from build123d import *

# Parameters (mm, degrees)
F0_R     = 2.3495
F0_R_2   = 9.525
F0_R_3   = 12.7
F0_R_4   = 2.0955
F0_R_5   = 10.9855
F1_DEPTH = 5
F2_R     = 19.05
F3_DEPTH = 5.08


with BuildPart() as f1:
    # F0 (on Top) → F1 (new body, symmetric)
    with BuildSketch(Plane.XY):
        with BuildLine():
            Line((-47.439466, 28.760534), (-44.025117, 25.346184))
            ThreePointArc((-44.025117, 25.346184), (-50.8, 0), (-44.025117, -25.346184))
            Line((-44.025117, -25.346184), (-47.439466, -28.760534))
            ThreePointArc((-47.439466, -28.760534), (-47.439466, -47.439466), (-28.760534, -47.439466))
            Line((-28.760534, -47.439466), (-25.346184, -44.025117))
            ThreePointArc((-25.346184, -44.025117), (0, -50.8), (25.346184, -44.025117))
            Line((25.346184, -44.025117), (28.760534, -47.439466))
            ThreePointArc((28.760534, -47.439466), (47.439466, -47.439466), (47.439466, -28.760534))
            Line((47.439466, -28.760534), (44.025117, -25.346184))
            ThreePointArc((44.025117, -25.346184), (50.8, 0), (44.025117, 25.346184))
            Line((44.025117, 25.346184), (47.439466, 28.760534))
            ThreePointArc((47.439466, 28.760534), (47.439466, 47.439466), (28.760534, 47.439466))
            Line((28.760534, 47.439466), (25.346184, 44.025117))
            ThreePointArc((25.346184, 44.025117), (0, 50.8), (-25.346184, 44.025117))
            Line((-25.346184, 44.025117), (-28.760534, 47.439466))
            ThreePointArc((-28.760534, 47.439466), (-47.439466, 47.439466), (-47.439466, 28.760534))
        make_face()
        with Locations((-41.304177, -41.314179)):
            Circle(F0_R, mode=Mode.SUBTRACT)
        with Locations((-36.206166, -0.017254)):
            Circle(F0_R_2, mode=Mode.SUBTRACT)
        with Locations((-25.384562, -25.40427)):
            Circle(F0_R_3, mode=Mode.SUBTRACT)
        with Locations((0.006088, -36.217333)):
            Circle(F0_R_2, mode=Mode.SUBTRACT)
        with Locations((41.314179, -41.304177)):
            Circle(F0_R, mode=Mode.SUBTRACT)
        with Locations((0, -14.605)):
            Circle(F0_R_4, mode=Mode.SUBTRACT)
        with Locations((25.40427, -25.384562)):
            Circle(F0_R_3, mode=Mode.SUBTRACT)
        with Locations((36.206166, -0.005079)):
            Circle(F0_R_2, mode=Mode.SUBTRACT)
        with Locations((-12.648301, 7.3025)):
            Circle(F0_R_4, mode=Mode.SUBTRACT)
        with Locations((-25.40427, 25.384562)):
            Circle(F0_R_3, mode=Mode.SUBTRACT)
        with Locations((-41.314179, 41.304177)):
            Circle(F0_R, mode=Mode.SUBTRACT)
        with Locations((-0.006088, 36.195)):
            Circle(F0_R_2, mode=Mode.SUBTRACT)
        Circle(F0_R_5, mode=Mode.SUBTRACT)
        with Locations((12.648301, 7.3025)):
            Circle(F0_R_4, mode=Mode.SUBTRACT)
        with Locations((25.384562, 25.40427)):
            Circle(F0_R_3, mode=Mode.SUBTRACT)
        with Locations((41.304177, 41.314179)):
            Circle(F0_R, mode=Mode.SUBTRACT)
    extrude(amount=F1_DEPTH, both=True)

    # F2 (on face) → F3 (cut)
    with BuildSketch(Plane.XY.offset(5)):
        Circle(F2_R)
    extrude(amount=-F3_DEPTH, mode=Mode.SUBTRACT)


solid = f1.part
Geometry check sheet. Reference: the model listing, model coordinates, mm. A direction names the side the tool comes from. Coordinates: 2 decimals unless noted, no trailing zeros. Order: outer loops, then holes, each group sorted by start corner. A loop starts at its lowest first (then second) coordinate and runs counter-clockwise, first axis right, second up. Notation, with made-up numbers: (-13.5, 0) -> (19.5, 0) arc R17 cw to (19.5, 5) -> close; hole circle Ø8 at (64.5, -21.75). An arc over 180 degrees is marked (long way). Use a Markdown table: item, result. Add a question column.
1. Cross-section at B-B (z = -3.75). Give the number of separate pieces and of enclosed holes in the cut face, and give its area (3 significant figures).
2. Material ranges on L1, parallel to Y at x = 2.5, z = -1.25; L2, parallel to X at y = 6, z = 1.5; L3, parallel to X at y = -23, z = 4, recorded low to high.
3. Set-up check for faces 5 (the face through (45.71, 27.03, 0.07)), 6 (the face through (27.08, 45.76, 0.07)), 7 (the face through (-15.12, -11.59, 2.5)), 8 (the face through (-45.76, 27.08, 0.07)): record each of +Z, -Z, +X, -X, +Y, -Y from which the full face is reachable in a straight line by a thin tool's end or side.
4. Cross-section at C-C (x = -24). Enter the section's corners in (y, z), and give its area (3 significant figures).
5. Mould release check, pull along Y, two halves, no side actions. Record for faces 1 (the face through (-27.03, 45.71, 0.07)), 2 (the face through (-1, 12, -5)), 3 (the face through (-0.4, -50.8, 0.1)), 4 (the face through (-1.25, 45.64, -0.07)): pulls with the +Y half, pulls with the -Y half, needs draft (parallel to the pull), parting line crosses it, or undercut.
6. Cross-section at A-A (x = 0). Enter the section's corners in (y, z), and give its area (3 significant figures).
7. Go/stop test with flat-tipped pins: pin 1 Ø2 at (x, z) = (6.5, 2) entering from +Y; pin 2 Ø4 at (y, z) = (22, -1) entering from -X; pin 3 Ø3 at (x, z) = (-1, 1) entering from +Y. Record where each tip stops, or that it passes through.
8. Cross-section at D-D (y = 32). Enter the section's corners in (x, z) (1 decimal), and give its area (3 significant figures).
Filled sheet:
| question | item | result |
|---|---|---|
| 1 | separate pieces | 1 |
| 1 | enclosed holes | 16 |
| 1 | area | 5,930 mm2 |
| 2 | L1 | -50.74 to -45.41, -27.02 to -10.7, 10.7 to 27.01, 45.38 to 50.74 |
| 2 | L2 | -50.44 to -43.59, -28.82 to -18.08, 18.08 to 28.81, 43.6 to 50.44 |
| 2 | L3 | -45.3 to -37.85, -12.91 to 12.93, 37.88 to 45.3 |
| 3 | face 5 | +Z, -Z, +X |
| 3 | face 6 | +Z, -Z, +Y |
| 3 | face 7 | +Z |
| 3 | face 8 | +Z, -Z, -X |
| 4 | outline | (-44.77, -5) -> (-38.03, -5) -> (-38.03, 5) -> (-44.77, 5) -> close; (-12.78, -5) -> (12.76, -5) -> (12.76, 5) -> (-12.78, 5) -> close; (38.01, -5) -> (44.77, -5) -> (44.77, 5) -> (38.01, 5) -> close |
| 4 | area | 391 mm2 |
| 5 | face 1 | pulls with the +Y half |
| 5 | face 2 | needs draft |
| 5 | face 3 | pulls with the -Y half |
| 5 | face 4 | undercut |
| 6 | outline | (-50.8, -5) -> (-45.74, -5) -> (-45.74, 5) -> (-50.8, 5) -> close; (-26.69, -5) -> (-16.7, -5) -> (-16.7, -0.08) -> (-19.05, -0.08) -> (-19.05, 5) -> (-26.69, 5) -> close; (-12.51, -5) -> (-10.99, -5) -> (-10.99, -0.08) -> (-12.51, -0.08) -> close; (10.99, -5) -> (26.67, -5) -> (26.67, 5) -> (19.05, 5) -> (19.05, -0.08) -> (10.99, -0.08) -> close; (45.72, -5) -> (50.8, -5) -> (50.8, 5) -> (45.72, 5) -> close |
| 6 | area | 313 mm2 |
| 7 | pin 1 | y = 50.5 |
| 7 | pin 2 | x = -46.7 |
| 7 | pin 3 | y = 50.8 |
| 8 | outline | (-49.8, -5) -> (-36.2, -5) -> (-36.2, 5) -> (-49.8, 5) -> close; (-14.6, -5) -> (-8.6, -5) -> (-8.6, 5) -> (-14.6, 5) -> close; (8.5, -5) -> (14.5, -5) -> (14.5, 5) -> (8.5, 5) -> close; (36.2, -5) -> (49.8, -5) -> (49.8, 5) -> (36.2, 5) -> close |
| 8 | area | 391 mm2 |
